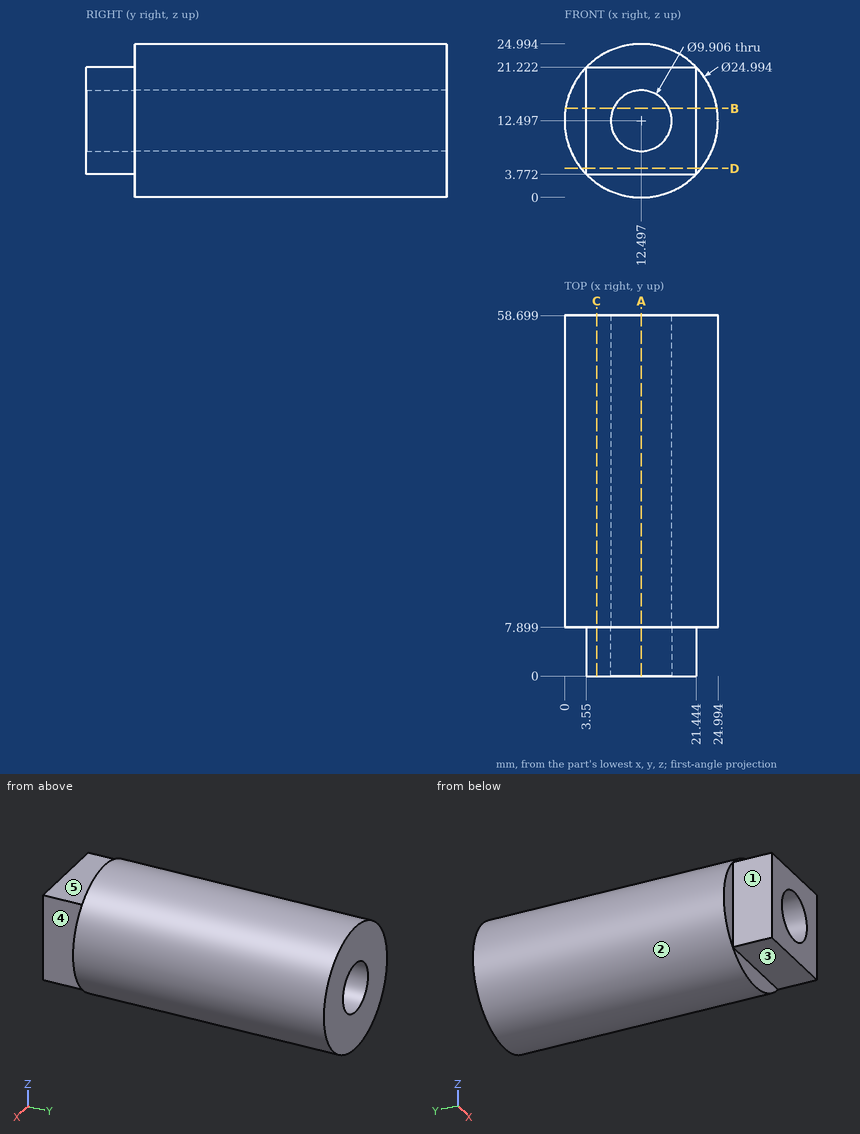
Print and shaded views of the part. All mm, measured from the part's lowest x, y and z. A direction names the side the tool comes from. Coordinates: 2 decimals unless noted, no trailing zeros. Order: outer loops, then holes, each group sorted by start corner. A loop starts at its lowest first (then second) coordinate and runs counter-clockwise, first axis right, second up. Notation, with made-up numbers: (65.25, 23) -> (84.25, 23) arc R22 cw to (84.25, 51) -> close; hole circle Ø9 at (63, 57). An arc over 180 degrees is marked (long way). Answer as a JSON object with one key per item and string values. Group by question number.
1) Which spindle directions (+Z, -Z, +X, -X, +Y, -Y) get a long thin tool onto all of the face, cutting with end or side? Do the marked faces 1, 2, 3, 4 and 5. Say none if no direction does.
2) Drill centre lines: L1, parallel to Y at x = 24, z = 17.25; L2, parallel to X at y = 29.5, z = 12 (1 decimal); L3, parallel to Z at x = 8.5, y = 55 (1 decimal). Where is each one in solid material? Low to high.
3) Cut at A-A, the plane x = 12.5. Write the cut outline in (y, z), then the cut area to 3 significant figures.
4) Cut at D-D, the plane z = 4.75. Write the cut outline in (x, y), then the cut area to 3 significant figures.
5) Cut at B-B, the plane z = 14.5. Write the cut outline in (x, y).
6) Flat gauge pins, fed straight in: pin 1 (2 mm diameter, centred on y = 22, z = 5.5, fed in from +X); pin 2 (3 mm diameter, centred on y = 47, z = 4.5, fed in from -X); pin 3 (8 mm diameter, centred on x = 12.5, z = 12.5, fed in from +Y); pin 4 (1.1 mm diameter, centred on x = 11, z = 1.5, fed in from -Y). Where does each tip first touch, or does it go through?
7) Cut at C-C, the plane x = 5.25. Write the cut outline in (y, z) (1 decimal), then the cut area to 3 significant figures.
Check values:
{
 "1": {"face 1": "+Z, -Z, -X, -Y", "face 2": "+Y, -Y", "face 3": "-Z, +X, -X, -Y", "face 4": "+Z, -Z, +X, -Y", "face 5": "+Z, +X, -X, -Y"},
 "2": {"L1": "y = 7.9 to 58.7", "L2": "x = 0 to 7.6, 17.4 to 25", "L3": "z = 0.7 to 9.6, 15.4 to 24.3"},
 "3": {"outline": "(0, 3.77) -> (7.9, 3.77) -> (7.9, 0) -> (58.7, 0) -> (58.7, 7.54) -> (0, 7.54) -> close; (0, 17.45) -> (58.7, 17.45) -> (58.7, 24.99) -> (7.9, 24.99) -> (7.9, 21.22) -> (0, 21.22) -> close", "area": "826 mm²"},
 "4": {"outline": "(2.69, 7.9) -> (3.55, 7.9) -> (3.55, 0) -> (21.44, 0) -> (21.44, 7.9) -> (22.3, 7.9) -> (22.3, 58.7) -> (2.69, 58.7) -> close", "area": "1,140 mm²"},
 "5": {"outline": "(0.16, 7.9) -> (3.55, 7.9) -> (3.55, 0) -> (7.97, 0) -> (7.97, 58.7) -> (0.16, 58.7) -> close; (17.03, 0) -> (21.44, 0) -> (21.44, 7.9) -> (24.83, 7.9) -> (24.83, 58.7) -> (17.03, 58.7) -> close"},
 "6": {"pin 1": "stops at x = 23.46", "pin 2": "stops at x = 1.82", "pin 3": "passes through", "pin 4": "stops at y = 7.9"},
 "7": {"outline": "(0, 3.8) -> (7.9, 3.8) -> (7.9, 2.3) -> (58.7, 2.3) -> (58.7, 22.7) -> (7.9, 22.7) -> (7.9, 21.2) -> (0, 21.2) -> close", "area": "1,170 mm²"}
}
